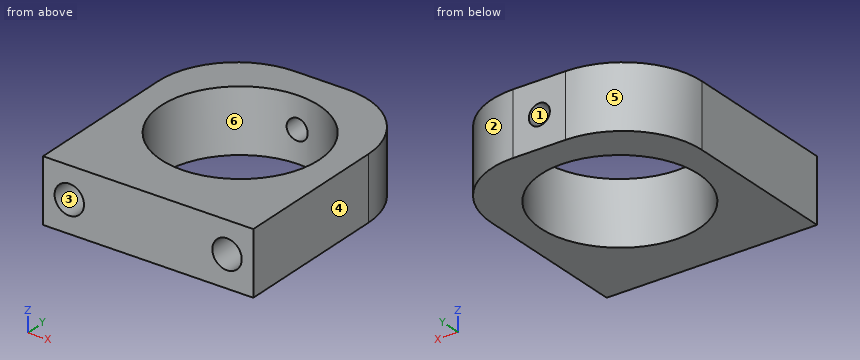
Autodesk Inventor part; units mm, degrees
ref_plane "YZ Plane" through (0, 0, 0) normal (1, 0, 0) x (0, 1, 0)
ref_plane "XZ Plane" through (0, 0, 0) normal (0, 1, 0) x (-1, 0, 0)
ref_plane "XY Plane" through (0, 0, 0) normal (0, 0, 1) x (1, 0, 0)
sketch "Skizze1" plane through (0, 0, 0) normal (0, 0, 1) x (1, 0, 0)
  line L0 (-20, -22.5) -> (20, -22.5)
  line L1 (20, -22.5) -> (20, 22.5)
  line L2 (20, 22.5) -> (-20, 22.5)
  line L3 (-20, 22.5) -> (-20, -22.5)
  line L4 (-20, -22.5) -> (20, 22.5) construction
  line L5 (20, -22.5) -> (-20, 22.5) construction
  point P0 (0, 0)
  dimension "d0" = 40
  dimension "d1" = 45
extrude "Extrusion1" add sketch "Skizze1" along normal mid plane 12
sketch "Skizze2" plane through (0, 0, 6) normal (0, 0, 1) x (1, 0, 0)
  circle A0 centre (0, 1.5) radius 15
  line L0 (20, 22.5) -> (-20, 22.5)
  point P0 (0, 0)
  point P1 (0, 22.5)
  dimension "d4" = 30
  dimension "d5" = 21
extrude "Extrusion2" cut sketch "Skizze2" against normal through all
sketch "Skizze3" plane through (-20, -22.5, 6) normal (0, -1, 0) x (1, 0, 0)
  line L0 (0, -12) -> (0, 0)
  line L1 (40, 0) -> (40, -12)
  point P0 (20, -6)
  point P1 (5, -6)
  point P2 (35, -6)
  dimension "d8" = 5
  dimension "d9" = 5
hole "Bohrung1" at (-15, -22.5, 0) at (15, -22.5, 0) direction (0, 1, 0) diameter 5.6 depth 11
sketch "Skizze4" plane through (-20, 22.5, 6) normal (0, 1, 0) x (1, 0, 0)
  point P0 (20, 6)
  point P1 (20, 6)
hole "Bohrung2" at (0, 22.5, 0) direction (0, -1, 0) diameter 4 depth 11
fillet "Rundung1" radius 15 2 edges at (-20, 22.5, 0) (20, 22.5, 0)
properties part number "FMR_DXWD80_CPW_Halter_B"
Work out the finished part from the listing and answer in its coordinate system (mm). Face numbers are marked on the shaded views. A direction names the side the tool comes from. Round coordinates to 2 decimals unless told otherwise and drop trailing zeros. Write each loop counter-clockwise with the first axis right and the second up, starting at its lowest first coordinate (ties: lowest second). Pieces come first, ordered by that corner, then holes. Notation, with made-up numbers: M 45.25,74.25 L 49.25,74.25 A23 cw 49.25,83.25 Z; hole C 2.5,-7 d8. An arc over 180 degrees is marked long. Use a Markdown table: item, result.
1) Determine the mould class of the marked faces 4, 5 and 6 for opening direction X: pulls with the +X half, pulls with the -X half, needs draft (parallel to the pull), parting line crosses it, or undercut.
Taken from the geometry:
| item | result |
|---|---|
| face 4 | pulls with the +X half |
| face 5 | pulls with the -X half |
| face 6 | undercut |
2) The part is cut by section B-B on y = 4.5. Give the vertices of the cut face in (x, z), plus the area to 3 significant figures.
Taken from the geometry:
| item | result |
|---|---|
| outline | M -20,-6 L -14.7,-6 L -14.7,6 L -20,6 Z; M 14.7,-6 L 20,-6 L 20,6 L 14.7,6 Z |
| area | 127 mm2 |
3) Consider line 1 (X direction, y = -18.5, z = 0); line 2 (Z direction, x = 15, y = -16); line 3 (Y direction, x = 4, z = 0.5). Determine where each line is inside the solid, lowest interval first. Write a range as [from, to].
Taken from the geometry:
| item | result |
|---|---|
| line 1 | x = [-20, -17.8], [-12.2, 12.2], [17.8, 20] |
| line 2 | z = [-6, -2.8], [2.8, 6] |
| line 3 | y = [-22.5, -12.96], [15.96, 22.5] |
4) Flat-ended cylindrical pins translate along their axes: pin 1 (3 mm diameter, centred on x = 14, z = -0.5, fed in from +Y); pin 2 (5 mm diameter, centred on x = -15, z = 0, fed in from -Y); pin 3 (2.5 mm diameter, centred on x = 0, z = 0, fed in from +Y). Find the tip coordinate at first contact, or state that the pin passes through.
Taken from the geometry:
| item | result |
|---|---|
| pin 1 | stops at y = 20.49 |
| pin 2 | stops at y = -11.5 |
| pin 3 | stops at y = -13.45 |
5) The part is cut by section D-D on x = 14. Give the vertices of the cut face in (y, z), plus the area to 3 significant figures.
Taken from the geometry:
| item | result |
|---|---|
| outline | M -22.5,-6 L -3.89,-6 L -3.89,6 L -22.5,6 L -22.5,2.62 L -11.5,2.62 L -11.5,-2.62 L -22.5,-2.62 Z; M 6.89,-6 L 19.5,-6 L 19.5,6 L 6.89,6 Z |
| area | 317 mm2 |
6) The part is cut by section A-A on x = 0. Give the vertices of the cut face in (y, z), plus the area to 3 significant figures.
Taken from the geometry:
| item | result |
|---|---|
| outline | M -22.5,-6 L -13.5,-6 L -13.5,6 L -22.5,6 Z; M 16.5,-6 L 22.5,-6 L 22.5,-2 L 16.5,-2 Z; M 16.5,2 L 22.5,2 L 22.5,6 L 16.5,6 Z |
| area | 156 mm2 |
7) The part is cut by section C-C on z = -4.75. Give the vertices of the cut face in (x, y), plus the area to 3 significant figures.
Taken from the geometry:
| item | result |
|---|---|
| outline | M -20,-22.5 L 20,-22.5 L 20,7.5 A15 ccw 5,22.5 L -5,22.5 A15 ccw -20,7.5 Z; hole C 0,1.5 d30 |
| area | 997 mm2 |
8) Which of the six approach directions +Z, -Z, +X, -X, +Y, -Y give full straight-line access (tool end or side, diameter ignored) to the marked faces 1, 2 and 3?
Taken from the geometry:
| item | result |
|---|---|
| face 1 | +Y |
| face 2 | +Z, -Z, +X, +Y |
| face 3 | -Y |
